```python
from build123d import *

# Parameters (mm, degrees)
F1_DEPTH = 57.15
F3_START = 12.7
F2_R     = 12.7
F3_DEPTH = 44.45
F5_START = 48.52348
F4_R     = 5.08
F5_DEPTH = 42.4313


with BuildPart() as f1:
    # F0 (on Front) → F1 (new body)
    with BuildSketch(Plane.XZ):
        Polygon((95.25, -8.89), (76.2, -8.89), (76.2, 0), (127, 0), (127, 63.5), (0, 63.5), (0, 0), (50.8, 0), (50.8, -8.89), (31.75, -8.89), (31.75, -21.59), (95.25, -21.59), align=None)
    extrude(amount=F1_DEPTH)

    # F2 (on Front) → F3 (cut)
    with BuildSketch(Plane.XZ.offset(F3_START)):
        with BuildLine():
            Line((127, 63.5), (65.383924195, 63.5))
            ThreePointArc((65.383924195, 63.5), (76.7139126522, 59.9653925056), (85.2011344437, 51.6690586863))
            Line((85.2011344437, 51.6690586863), (111.125, 12.7))
            Line((111.125, 12.7), (127, 12.7))
            Line((127, 12.7), (127, 63.5))
        make_face()
        with BuildLine():
            ThreePointArc((65.383924195, 63.5), (63.693806529, 63.5562926494), (62.0036888631, 63.5))
            Line((62.0036888631, 63.5), (65.383924195, 63.5))
        make_face()
        with BuildLine():
            Line((62.0036888631, 63.5), (0, 63.5))
            Line((0, 63.5), (0, 12.7))
            Line((0, 12.7), (15.875, 12.7))
            Line((15.875, 12.7), (42.0723728562, 51.485718966))
            ThreePointArc((42.0723728562, 51.485718966), (50.5811087271, 59.9098476773), (62.0036888631, 63.5))
        make_face()
        with Locations((63.693806529, 38.1562926494)):
            Circle(F2_R)
    extrude(amount=F3_DEPTH, mode=Mode.SUBTRACT)

    # F4 (on Top) → F5 (cut)
    with BuildSketch(Plane.XY.offset(F5_START)):
        with Locations((63.5088086128, -34.925)):
            Circle(F4_R)
    extrude(amount=F5_DEPTH, mode=Mode.SUBTRACT)


solid = f1.part
```
Read the model definition and answer for the solid it produces. Units are mm, in the model's axes. A direction names the side the tool comes from. Give positions to 0.01 mm unless a question says otherwise; leave off trailing zeros. Order: outer loops, then holes, each group sorted by start corner. A loop starts at its lowest first (then second) coordinate and runs counter-clockwise, first axis right, second up. Notation, with made-up numbers: (69, 49.5) -> (124, 49.5) arc R15 cw to (124, 72.5) -> close; hole circle Ø9 at (-20, 89.5). An arc over 180 degrees is marked (long way). Write item = value, one per line.
1. For faces 4 (the face through (31.75, -28, -15)), 5 (the face through (50.8, -28, -4)), 6 (the face through (109, -12.7, 44)), 7 (the face through (8, -35, 12.7)), determine the directions among +Z, -Z, +X, -X, +Y, -Y from which every point of the face is accessible in a straight line to the end or side of a thin tool.
Numbers:
face_4 = -Z, -X, +Y, -Y
face_5 = -X, +Y, -Y
face_6 = +Z, +X, -Y
face_7 = +Z, -X, -Y
2. A cutting plane is placed at D-D, the plane y = -48.5. Write down the section's boundary in (x, z) (3 decimals), and give its area (3 significant figures).
Numbers:
outline = (0, 0) -> (50.8, 0) -> (50.8, -8.89) -> (31.75, -8.89) -> (31.75, -21.59) -> (95.25, -21.59) -> (95.25, -8.89) -> (76.2, -8.89) -> (76.2, 0) -> (127, 0) -> (127, 12.7) -> (111.125, 12.7) -> (85.201, 51.669) arc R25.4 ccw to (65.384, 63.5) -> (62.004, 63.5) arc R25.4 ccw to (42.072, 51.486) -> (15.875, 12.7) -> (0, 12.7) -> close; hole circle Ø25.4 at (63.694, 38.156)
area = 5,190 mm²
3. A cutting plane is placed at C-C, the plane x = 12.5. Write down the section's boundary in (y, z), and give its area (3 significant figures).
Numbers:
outline = (-57.15, 0) -> (0, 0) -> (0, 63.5) -> (-12.7, 63.5) -> (-12.7, 12.7) -> (-57.15, 12.7) -> close
area = 1,370 mm²
4. The mould has two halves that part along Z. Classify faces 1 (the face through (28.79, -34.61, 31.82)), 2 (the face through (60.94, -34.61, 25.76)), 3 (the face through (0, -9, 18)): +Z half, -Z half, draft (parallel to the pull), parting line (faces both ways), or undercut.
Numbers:
face_1 = +Z half
face_2 = undercut
face_3 = draft
5. A cutting plane is placed at B-B, the plane x = 89. Write down the section's boundary in (y, z), and give its area (3 significant figures).
Numbers:
outline = (-57.15, -21.59) -> (0, -21.59) -> (0, -8.89) -> (-57.15, -8.89) -> close; (-57.15, 0) -> (0, 0) -> (0, 63.5) -> (-12.7, 63.5) -> (-12.7, 45.96) -> (-57.15, 45.96) -> close
area = 3,580 mm²
6. Given pin 1 (2.5 mm diameter, centred on y = -19, z = -4, fed in from +X); pin 2 (8 mm diameter, centred on x = 120, y = -31.5, fed in from +Z); pin 3 (2 mm diameter, centred on x = 100, y = -31, fed in from +Z), each flat-ended and moving along its own axis, determine where each tip first touches the part or whether it passes through.
Numbers:
pin_1 = 76.2
pin_2 = 12.7
pin_3 = 30.93
7. A cutting plane is placed at A-A, the plane y = -5. Write down the section's boundary in (x, z).
Numbers:
outline = (0, 0) -> (50.8, 0) -> (50.8, -8.89) -> (31.75, -8.89) -> (31.75, -21.59) -> (95.25, -21.59) -> (95.25, -8.89) -> (76.2, -8.89) -> (76.2, 0) -> (127, 0) -> (127, 63.5) -> (0, 63.5) -> close
8. Straight lines are drawn through the part: line 1 along Y through (x, z) = (24, 52); line 2 along Z through (x, y) = (48, -10.5); line 3 along X through (y, z) = (-46, 41). For each, find the intervals that lie inside material, in ascending order.
Numbers:
line_1 = -12.7 to 0
line_2 = -21.59 to -8.89, 0 to 63.5
line_3 = 34.99 to 51.32, 76.07 to 92.3
